The model under review builds one solid part; all positions refer to its coordinate system, in mm. Coordinates: 2 decimals unless noted, no trailing zeros. Write each loop counter-clockwise with the first axis right and the second up, starting at its lowest first coordinate (ties: lowest second). Pieces come first, ordered by that corner, then holes. Notation, with made-up numbers: (24.5, 29.25) -> (39.5, 29.25) arc R22 cw to (39.5, 46.25) -> close; hole circle Ø11 at (88.5, -17.75). An arc over 180 degrees is marked (long way). Write each question's results on one line, items separated by ' | '.
Autodesk Inventor part; units mm, degrees
ref_plane "YZ Plane" through (0, 0, 0) normal (1, 0, 0) x (0, 1, 0)
ref_plane "XZ Plane" through (0, 0, 0) normal (0, 1, 0) x (-1, 0, 0)
ref_plane "XY Plane" through (0, 0, 0) normal (0, 0, 1) x (1, 0, 0)
sketch "Szkic1" plane through (0, 0, 0) normal (0, 0, 1) x (1, 0, 0)
  line L0 (-20.451, -12.8135) -> (535.549, -12.8135)
  line L1 (535.549, -12.8135) -> (535.549, 159.1865)
  line L2 (515.549, 179.1865) -> (419.549, 179.1865)
  line L3 (399.549, 159.1865) -> (399.549, 104.1865)
  line L4 (374.549, 79.1865) -> (-20.451, 79.1865)
  line L5 (-20.451, 79.1865) -> (-20.451, -12.8135)
  line L6 (419.049, 155.1865) -> (494.049, 155.1865)
  line L7 (494.049, 155.1865) -> (494.049, 112.1865)
  line L8 (494.049, 112.1865) -> (419.049, 112.1865)
  line L9 (419.049, 112.1865) -> (419.049, 155.1865)
  arc A0 (374.549, 79.1865) -> (399.549, 104.1865) centre (374.549, 104.1865) ccw
  arc A1 (419.549, 179.1865) -> (399.549, 159.1865) centre (419.549, 159.1865) ccw
  arc A2 (535.549, 159.1865) -> (515.549, 179.1865) centre (515.549, 159.1865) ccw
  circle A3 centre (493.049, 90.1865) radius 8
  circle A4 centre (475.049, 90.1865) radius 2.5
  circle A5 centre (459.849, 90.1865) radius 2.5
  circle A6 centre (189.549, 28.1865) radius 11
  circle A7 centre (129.549, 28.1865) radius 11
  circle A8 centre (59.549, 28.1865) radius 11
  point P0 (0, 0)
  point P1 (535.549, 179.1865)
  point P2 (399.549, 179.1865)
  point P3 (399.549, 79.1865)
  point P4 (500.549, 166.1865)
  point P5 (500.549, 101.1865)
  point P6 (412.549, 101.1865)
  point P7 (412.549, 166.1865)
  point P8 (386.049, 62.1865)
  point P9 (522.049, 164.1865)
  point P10 (522.049, 2.1865)
  point P11 (-6.951, 2.1865)
  point P12 (-6.951, 62.1865)
  point P13 (189.549, 62.1865)
  dimension "d0" = 556
  dimension "d1" = 92
  dimension "d2" = 100
  dimension "d3" = 136
  dimension "d6" = 75
  dimension "d7" = 43
  dimension "d8" = 24
  dimension "d12" = 25
  dimension "d13" = 20
  dimension "d14" = 20
  dimension "d15" = 41.5
  dimension "d18" = 6.5
  dimension "d19" = 6.5
  dimension "d20" = 6.5
  dimension "d21" = 6.5
  dimension "d22" = 11
  dimension "d23" = 11
  dimension "d24" = 11
  dimension "d25" = 11
  dimension "d33" = 16
  dimension "d34" = 5
  dimension "d35" = 5
  dimension "d40" = 18
  dimension "d41" = 15.2
  dimension "d44" = 13.5
  dimension "d45" = 13.5
  dimension "d46" = 13.5
  dimension "d47" = 13.5
  dimension "d48" = 17
  dimension "d49" = 17
  dimension "d50" = 17
  dimension "d58" = 15
  dimension "d59" = 15
  dimension "d60" = 15
  dimension "d61" = 13.5
  dimension "d62" = 393
  dimension "d63" = 196.5
  dimension "d64" = 22
  dimension "d65" = 22
  dimension "d66" = 22
  dimension "d67" = 41
  dimension "d68" = 41
  dimension "d69" = 41
  dimension "d71" = 70
  dimension "d72" = 60
  dimension "d73" = 80
  dimension "d74" = 88
  dimension "d75" = 65
  dimension "d79" = 65
  dimension "d80" = 7.5
  dimension "d81" = 11
  dimension "d82" = 11
  dimension "d83" = 11
extrude "Wyciągnięcie proste2" add sketch "Szkic1" along normal blind 2 contours L5 L4 A0 L3 A1 L2 A2 L1 L0 | A3 | A4 | A5 | A6 | A7 | A8
fillet "Zaokrąglenie1" radius 2 4 edges at (419.049, 112.1865, 1) (494.049, 112.1865, 1) (494.049, 155.1865, 1) (419.049, 155.1865, 1)
hole "Otwór1" at (500.549, 166.1865, 0) at (500.549, 101.1865, 0) at (412.549, 101.1865, 0) at (412.549, 166.1865, 0) direction (0, 0, 1) diameter 3 end through all
extrude "Wyciągnięcie proste3" cut sketch "Szkic1" along normal blind 10 contours A3 | A4 | A5 | A6 | A7 | A8
hole "Otwór2" at (386.049, 62.1865, 0) at (522.049, 164.1865, 0) at (522.049, 2.1865, 0) at (-6.951, 2.1865, 0) at (-6.951, 62.1865, 0) at (189.549, 62.1865, 0) direction (0, 0, 1) diameter 4 end through all
equation "\"d68\" = d67"
equation "\"d69\" = d67"
properties part number "LC_ALU_2mm_Front_Plate"
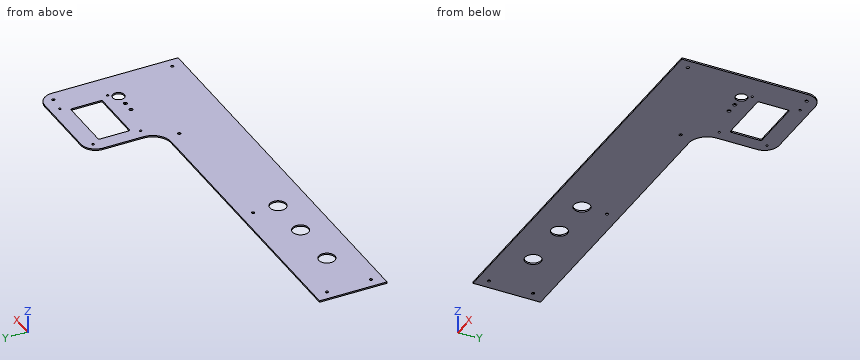
Q1. Clearance check with flat-ended pins moving along their axes: P1, Ø4, axis at x = 412.55, y = 166.19, coming from the +Z side; P2, Ø17.5, axis at x = 59.55, y = 28.19, coming from the +Z side. State where each tip first meets the part, or that it passes through.
Solution:
P1: z = 2 | P2: through
Q2. Add section C-C (x = 321.5). Write out the cut boundary in (y, z).
Solution:
outline: (-12.81, 0) -> (79.19, 0) -> (79.19, 2) -> (-12.81, 2) -> close
Q3. For line 1 (Y direction, x = 449.5, z = 0.15); line 2 (X direction, y = 2.5, z = 0.15); line 3 (X direction, y = 121.5, z = 0.85), list the stretches that pass through material, from the lowest coordinate up. Write a range as from..to.
Solution:
line 1: -12.81..112.19, 155.19..179.19 | line 2: -20.45..-8.93, -4.98..520.07, 524.02..535.55 | line 3: 399.55..419.05, 494.05..535.55
Q4. Add section B-B (z = 1.65). Count the separate pieces of the cut face and the enclosed holes in it, plus the area to 3 significant figures.
Solution:
separate pieces: 1 | enclosed holes: 17 | area: 60,000 mm²
Q5. Add section A-A (y = 121). Write out the cut boundary in (x, z), plus the area to 3 significant figures.
Solution:
outline: (399.55, 0) -> (419.05, 0) -> (419.05, 2) -> (399.55, 2) -> close; (494.05, 0) -> (535.55, 0) -> (535.55, 2) -> (494.05, 2) -> close | area: 122 mm²
